from build123d import *

# Parameters (mm, degrees)
SKETCH_1_R          = 21.5
SKETCH_1_R_2        = 2.1
SKETCH_1_W          = 4
SKETCH_1_H          = 1.5
EXTRUDE_1_DEPTH     = 4
SKETCH_3_R          = 1.5
SKETCH_3_R_2        = 1.65
SKETCH_3_W          = 8.03
SKETCH_3_H          = 4.03
SKETCH_3_W_2        = 4.03
SKETCH_3_H_2        = 8.03
CUT_EXTRUDE_2_DEPTH = 4
SKETCH_7_R          = 3
CUT_EXTRUDE_3_DEPTH = 10
SKETCH_8_W          = 220
SKETCH_8_H          = 220
CUT_EXTRUDE_4_DEPTH = 4


with BuildPart() as part:
    # 草图1 → 凸台-拉伸1 (new body)
    with BuildSketch(Plane.XY):
        Polygon((151.457142857, -41.187142857), (151.457142857, 108.812857143), (-148.542857143, 108.812857143), (-148.542857143, -191.187142857), (151.457142857, -191.187142857), align=None)
        with Locations((1.457142857, -41.187142857)):
            Circle(SKETCH_1_R, mode=Mode.SUBTRACT)
        with Locations((25.027142857, -17.617142857)):
            Circle(SKETCH_1_R_2, mode=Mode.SUBTRACT)
        with Locations((25.027142857, -64.757142857)):
            Circle(SKETCH_1_R_2, mode=Mode.SUBTRACT)
        with Locations((-22.112857143, -64.757142857)):
            Circle(SKETCH_1_R_2, mode=Mode.SUBTRACT)
        with Locations((-22.112857143, -17.617142857)):
            Circle(SKETCH_1_R_2, mode=Mode.SUBTRACT)
        with Locations((65.457142857, 98.062857143)):
            Rectangle(SKETCH_1_W, SKETCH_1_H, mode=Mode.SUBTRACT)
        with Locations((-62.542857143, 98.062857143)):
            Rectangle(SKETCH_1_W, SKETCH_1_H, mode=Mode.SUBTRACT)
    extrude(amount=EXTRUDE_1_DEPTH)

    # 草图3 → 切除-拉伸2 (cut)
    with BuildSketch(Plane.XY.offset(4)):
        with Locations((1.457142857, -185.187142857)):
            Circle(SKETCH_3_R)
        with Locations((67.457142857, -185.187142857)):
            Circle(SKETCH_3_R)
        with Locations(Location((-64.542857143, -185.187142857, 0), (0, 0, 180))):
            Circle(SKETCH_3_R)
        with Locations(Location((-142.542857143, 24.812857143, 0), (0, 0, 180))):
            Circle(SKETCH_3_R)
        with Locations((-142.542857143, -41.187142857)):
            Circle(SKETCH_3_R)
        with Locations((-142.542857143, -107.187142857)):
            Circle(SKETCH_3_R)
        with Locations(Location((67.457142857, 102.812857143, 0), (0, 0, 180))):
            Circle(SKETCH_3_R)
        with Locations((1.457142857, 102.812857143)):
            Circle(SKETCH_3_R)
        with Locations((-64.542857143, 102.812857143)):
            Circle(SKETCH_3_R)
        with Locations(Location((145.457142857, -107.187142857, 0), (0, 0, 180))):
            Circle(SKETCH_3_R)
        with Locations((145.457142857, -41.187142857)):
            Circle(SKETCH_3_R)
        with Locations((145.457142857, 24.812857143)):
            Circle(SKETCH_3_R)
        with Locations((1.457142857, -108.687142857)):
            Circle(SKETCH_3_R_2)
        with Locations((-46.272564873, -88.916850587)):
            Circle(SKETCH_3_R_2)
        with Locations((-66.042857143, -41.187142857)):
            Circle(SKETCH_3_R_2)
        with Locations((-46.272564873, 6.542564873)):
            Circle(SKETCH_3_R_2)
        with Locations((1.457142857, 26.312857143)):
            Circle(SKETCH_3_R_2)
        with Locations((49.186850587, 6.542564873)):
            Circle(SKETCH_3_R_2)
        with Locations((68.957142857, -41.187142857)):
            Circle(SKETCH_3_R_2)
        with Locations((49.186850587, -88.916850587)):
            Circle(SKETCH_3_R_2)
        with Locations((1.457142857, -125.187142857)):
            Circle(SKETCH_3_R)
        with Locations((100.457142857, -185.187142857)):
            Rectangle(SKETCH_3_W, SKETCH_3_H)
        with Locations((34.457142857, -185.187142857)):
            Rectangle(SKETCH_3_W, SKETCH_3_H)
        with Locations((-31.542857143, -185.187142857)):
            Rectangle(SKETCH_3_W, SKETCH_3_H)
        with Locations((-97.542857143, -185.187142857)):
            Rectangle(SKETCH_3_W, SKETCH_3_H)
        with Locations((-142.542857143, 57.812857143)):
            Rectangle(SKETCH_3_W_2, SKETCH_3_H_2)
        with Locations((-142.542857143, -8.187142857)):
            Rectangle(SKETCH_3_W_2, SKETCH_3_H_2)
        with Locations((-142.542857143, -74.187142857)):
            Rectangle(SKETCH_3_W_2, SKETCH_3_H_2)
        with Locations((-142.542857143, -140.187142857)):
            Rectangle(SKETCH_3_W_2, SKETCH_3_H_2)
        with Locations((100.457142857, 102.812857143)):
            Rectangle(SKETCH_3_W, SKETCH_3_H)
        with Locations((34.457142857, 102.812857143)):
            Rectangle(SKETCH_3_W, SKETCH_3_H)
        with Locations((-31.542857143, 102.812857143)):
            Rectangle(SKETCH_3_W, SKETCH_3_H)
        with Locations((-97.542857143, 102.812857143)):
            Rectangle(SKETCH_3_W, SKETCH_3_H)
        with Locations((145.457142857, -140.187142857)):
            Rectangle(SKETCH_3_W_2, SKETCH_3_H_2)
        with Locations((145.457142857, -74.187142857)):
            Rectangle(SKETCH_3_W_2, SKETCH_3_H_2)
        with Locations((145.457142857, -8.187142857)):
            Rectangle(SKETCH_3_W_2, SKETCH_3_H_2)
        with Locations((145.457142857, 57.812857143)):
            Rectangle(SKETCH_3_W_2, SKETCH_3_H_2)
    extrude(amount=-CUT_EXTRUDE_2_DEPTH, mode=Mode.SUBTRACT)

    # 草图7 → 切除-拉伸3 (cut)
    with BuildSketch(Plane.XY.offset(4)):
        with Locations((-88.542857143, -171.187142857)):
            Circle(SKETCH_7_R)
        with Locations((91.457142857, -171.187142857)):
            Circle(SKETCH_7_R)
        with Locations((-128.542857143, 48.812857143)):
            Circle(SKETCH_7_R)
        with Locations((-128.542857143, -131.187142857)):
            Circle(SKETCH_7_R)
        with Locations((91.457142857, 88.812857143)):
            Circle(SKETCH_7_R)
        with Locations((-88.542857143, 88.812857143)):
            Circle(SKETCH_7_R)
        with Locations((131.457142857, -131.187142857)):
            Circle(SKETCH_7_R)
        with Locations((131.457142857, 48.812857143)):
            Circle(SKETCH_7_R)
    extrude(amount=-CUT_EXTRUDE_3_DEPTH, mode=Mode.SUBTRACT)

    # 草图8 → 切除-拉伸4 (cut)
    with BuildSketch(Plane.XY.offset(4)):
        with Locations((1.457142857, -41.187142857)):
            Rectangle(SKETCH_8_W, SKETCH_8_H)
    extrude(amount=-CUT_EXTRUDE_4_DEPTH, mode=Mode.SUBTRACT)


solid = part.part
Source: CAD feature listing. Evaluate the final solid. Frame: model axes, mm. Round coordinates to 2 decimals unless told otherwise and drop trailing zeros. Loops run counter-clockwise (first coordinate to the right, second up) from the corner with the lowest first, then second, coordinate; pieces in that order, holes last. Notation, with made-up numbers: (-34.75, 87.5) - (-25.75, 87.5) arc R19 ccw to (-25.75, 118.5) - close; hole circle Ø2 at (69, 14.5). An arc over 180 degrees is marked (long way). Write item = value, one per line. Start each with the question number.
(1) Section query A-A, the plane x = -31. Output: boundary loops of the cut face in (y, z).
(2) Section query D-D, the plane z = 0.8. State how many separate pieces and enclosed holes the cut face has, plus the area to 3 significant figures.
(3) Section query C-C, the plane x = 11. Output: boundary loops of the cut face in (y, z).
(4) Section query B-B, the plane y = -27. Output: boundary loops of the cut face in (x, z), plus the area to 3 significant figures.
(5) Pin query (flat end, axial travel): pin 1 (12 mm diameter, centred on x = 109, y = 13, fed in from +Z). Return the tip coordinate at first contact, or that it passes through.
(6) Ray query, line 1 along X through (y, z) = (58, 3.35); line 2 along Y through (x, z) = (-89, 3.25); line 3 along X through (y, z) = (-44, 2.45). Return the intervals inside material, ascending. Write a range as from..to.
Conclusion:
q1.outline = (-191.19, 0) - (-187.2, 0) - (-187.2, 4) - (-191.19, 4) - close; (-183.17, 0) - (-151.19, 0) - (-151.19, 4) - (-183.17, 4) - close; (68.81, 0) - (100.8, 0) - (100.8, 4) - (68.81, 4) - close; (104.83, 0) - (108.81, 0) - (108.81, 4) - (104.83, 4) - close
q2.separate_pieces = 1
q2.enclosed_holes = 39
q2.area = 40,800 mm2
q3.outline = (-191.19, 0) - (-151.19, 0) - (-151.19, 4) - (-191.19, 4) - close; (68.81, 0) - (108.81, 0) - (108.81, 4) - (68.81, 4) - close
q4.outline = (-148.54, 0) - (-108.54, 0) - (-108.54, 4) - (-148.54, 4) - close; (111.46, 0) - (151.46, 0) - (151.46, 4) - (111.46, 4) - close
q4.area = 320 mm2
q5.pin_1 = 4
q6.line_1 = -148.54..-144.56, -140.53..-108.54, 111.46..143.44, 147.47..151.46
q6.line_2 = -191.19..-174.15, -168.22..-151.19, 68.81..85.85, 91.78..108.81
q6.line_3 = -148.54..-108.54, 111.46..151.46
